from build123d import *

# Parameters (mm, degrees)
SKETCH1_W                      = 40
SKETCH1_H                      = 40
BOSS_EXTRUDE1_DEPTH            = 22
SKETCH2_W                      = 20.5
SKETCH2_H                      = 38.5
CUT_EXTRUDE1_DEPTH             = 60.896458739
M24_CLEARANCE_HOLE1_D          = 26.7
M24_CLEARANCE_HOLE1_DEPTH      = 4.972963553
F_3_3_3_3_DIAMETER_HOLE1_D     = 3.3
F_3_3_3_3_DIAMETER_HOLE1_DEPTH = 4.972963553
F_3_0_3_DIAMETER_HOLE1_D       = 3
FILLET1_R                      = 1.5
FILLET2_R                      = 2
FILLET3_R                      = 3
FILLET4_R                      = 10


with BuildPart() as part:
    # Sketch1 → Boss-Extrude1 (new body)
    with BuildSketch(Plane(origin=(-1.395486846, 0, 15.950487634), x_dir=(0, -1, 0), z_dir=(-0.08715574274765787, 0, 0.9961946980917457))):
        with Locations((-20.4, -0.261467228)):
            Rectangle(SKETCH1_W, SKETCH1_H)
    extrude(amount=-BOSS_EXTRUDE1_DEPTH)

    # Sketch2 → Cut-Extrude1 (cut, through all)
    with BuildSketch(Plane(origin=(19.663421695, 0, 1.720326484), x_dir=(0.08715574274765787, 0, -0.9961946980917455), z_dir=(0.9961946980917455, 3.832107347333544e-15, 0.08715574274765787))):
        with Locations((-5.761415906, 19.65)):
            Rectangle(SKETCH2_W, SKETCH2_H)
    extrude(amount=-CUT_EXTRUDE1_DEPTH, mode=Mode.SUBTRACT)

    # M24 Clearance Hole1
    with Locations(Plane(origin=(0.391205881, 0, -4.471503677), x_dir=(0.9961946980917455, 0, 0.08715574274765787), z_dir=(-0.08715574274765787, 0, 0.9961946980917455))):
        with Locations((-0.261467228, 20.2)):
            Hole(M24_CLEARANCE_HOLE1_D / 2, depth=M24_CLEARANCE_HOLE1_DEPTH)

    # Ø3.3 (3.3) Diameter Hole1
    with Locations(Plane(origin=(0.391205881, 0, -4.471503677), x_dir=(0.9961946980917455, 0, 0.08715574274765787), z_dir=(-0.08715574274765787, 0, 0.9961946980917455))):
        with Locations((-0.261467228, 4.95), (-7.886467228, 6.993112592), (-13.468354636, 12.575), (-15.511467228, 20.2), (-13.468354636, 27.825), (-7.886467228, 33.406887408), (-0.261467228, 35.45), (7.363532772, 33.406887408), (12.945420179, 27.825), (14.988532772, 20.2), (12.945420179, 12.575), (7.363532772, 6.993112592)):
            Hole(F_3_3_3_3_DIAMETER_HOLE1_D / 2, depth=F_3_3_3_3_DIAMETER_HOLE1_DEPTH)

    # Ø3.0 (3) Diameter Hole1 (through all)
    with Locations(Plane(origin=(0, 38.9, 0), x_dir=(-1, 0, 0), z_dir=(0, -1, 0))):
        with Locations((-14.651558368, -0.490248903), (-14.128623911, -6.467417091), (-13.605689455, -12.44458528), (15.035043636, 2.106992231), (15.557978092, -3.870175957), (16.080912549, -9.847344146)):
            Hole(F_3_0_3_DIAMETER_HOLE1_D / 2)

    # Fillet1
    fillet1_edges = [part.edges().sort_by_distance(p)[0] for p in [
        (0.130733614, 38.9, -4.494292047),
    ]]
    fillet(fillet1_edges, radius=FILLET1_R)

    # Fillet2
    fillet2_edges = [part.edges().sort_by_distance(p)[0] for p in [
        (18.26793485, 39.65, 17.670814119),
        (-21.579853074, 39.65, 14.184584409),
    ]]
    fillet(fillet2_edges, radius=FILLET2_R)

    # Fillet3
    fillet3_edges = [part.edges().sort_by_distance(p)[0] for p in [
        (0.261467228, 40.4, -5.988584094),
    ]]
    fillet(fillet3_edges, radius=FILLET3_R)

    # Fillet4
    fillet4_edges = [part.edges().sort_by_distance(p)[0] for p in [
        (20.119994383, 0.4, -3.498323216),
        (-19.727793541, 0.4, -6.984552926),
    ]]
    fillet(fillet4_edges, radius=FILLET4_R)


solid = part.part
Source: CAD feature listing. Evaluate the final solid. Frame: model axes, mm. A direction names the side the tool comes from. Round coordinates to 2 decimals unless told otherwise and drop trailing zeros. Write each loop counter-clockwise with the first axis right and the second up, starting at its lowest first coordinate (ties: lowest second). Pieces come first, ordered by that corner, then holes. Notation, with made-up numbers: (80, 12) - (135, 12) arc R8 cw to (135, 20) - close; hole circle Ø2 at (-20, -23.5). An arc over 180 degrees is marked (long way). Use CSV: the item, a comma, the result in double quotes. Start each with the question number.
(1) Cut plane A-A, the plane y = 25.5. Return loops of the section in (x, z).
(2) Cut plane C-C, the plane x = 1. Give the number of separate pieces and of enclosed holes in the cut face, and give its area (3 significant figures).
(3) First-contact query: pin 1 Ø2 at (x, y) = (14, 9.5) entering from +Z; pin 2 Ø6.5 at (x, z) = (-2, 11.5) entering from -Y; pin 3 Ø10 at (x, y) = (1, 5) entering from -Z; pin 4 Ø1.8 at (x, z) = (13.61, 12.44) entering from -Y. Flat tips, straight axial feed; report the tip coordinate or a pass-through.
(4) Material intervals for probe 1 along Y at (x, z) = (17, 12.5); probe 2 along Z at (x, y) = (18.5, 36.5); probe 3 along Z at (x, y) = (-19, 7.5), sorted ascending. Write a range as [from, to].
(5) Cut plane B-B, the plane y = 8. Return loops of the section in (x, z).
(6) Cut plane D-D, the plane y = 18. Return loops of the section in (x, z), and give its area (3 significant figures).
(7) Mould query, pull axis Z, two halves, no side actions, for faces 1 (the face through (17.72, 39.64, 17.05)), 2 (the face through (13.823, 19.159, -4.802)), 3 (the face through (12.63, 39.66, 6.4)). Classes: pulls with the +Z half, pulls with the -Z half, needs draft (parallel to the pull), parting line crosses it, or undercut.
(8) Set-up query: faces 4 (the face through (4.837, 6.308, -4.083)), 5 (the face through (-16.89, 3.41, -6.75)). Return all of +Z, -Z, +X, -X, +Y, -Y with unobstructed straight access to the full face (end or side cutting, diameter ignored); none if empty.
Geometry says:
1,outline,"(-19.79, -6.24) - (-19.66, -7.73) - (-11.94, -7.06) - (-12.08, -5.56) - close; (12.34, -3.43) - (12.47, -4.92) - (20.19, -4.25) - (20.05, -2.75) - close"
2,separate pieces,"4"
2,enclosed holes,"0"
2,area,"40.8 mm²"
3,pin 1,"z = -3.19"
3,pin 2,"y = 38.9"
3,pin 3,"z = -6.36"
3,pin 4,"through"
4,probe 1,"[38.9, 40.4]"
4,probe 2,"[-4.39, -2.89]"
4,probe 3,"[-7.67, -6.17]"
5,outline,"(-19.5, -6.21) - (-19.37, -7.71) - (-8.64, -6.77) - (-8.77, -5.27) - close; (-6.16, -5.04) - (-6.03, -6.54) - (-5.14, -6.46) - (-5.27, -4.97) - close; (5.53, -4.02) - (5.66, -5.52) - (6.56, -5.44) - (6.42, -3.94) - close; (9.03, -3.72) - (9.16, -5.21) - (19.89, -4.27) - (19.76, -2.78) - close"
6,outline,"(-19.79, -6.24) - (-19.66, -7.73) - (-12.86, -7.14) - (-12.99, -5.64) - close; (13.25, -3.35) - (13.38, -4.84) - (20.19, -4.25) - (20.05, -2.75) - close"
6,area,"20.5 mm²"
7,face 1,"pulls with the +Z half"
7,face 2,"pulls with the -Z half"
7,face 3,"undercut"
8,face 4,"+Z, -X, -Y"
8,face 5,"-Z, -X, -Y"
